from build123d import *

# Parameters (mm, degrees)
F1_DEPTH = 5.1
F2_W     = 3.2
F2_H     = 3.2
F4_DEPTH = 11
F3_W     = 3.2
F3_H     = 3.2
F5_DEPTH = 11
F6_DEPTH = 1


# Not quite as in the source:
# - a feature names something its author has since deleted; it is built from what else it names


with BuildPart() as f1:
    # F0 (on Top) → F1 (new body)
    with BuildSketch(Plane.XY):
        Polygon((-17.8524617243, -0.2032842353), (-25.3224617243, -0.2032842353), (-25.3224617243, -13.2032842353), (-5.3224617243, -13.2032842353), (-5.3224617243, -0.2032842353), (-12.7924617243, -0.2032842353), (-12.7924617243, -8.0232842353), (-11.6424617243, -8.0232842353), (-11.6424617243, -10.1232842353), (-19.0024617243, -10.1232842353), (-19.0024617243, -8.0232842353), (-17.8524617243, -8.0232842353), align=None)
    extrude(amount=F1_DEPTH)

    # F2 (on face) → F4 (cut)
    with BuildSketch(Plane(origin=(0, -0.2032842353, 0), x_dir=(-1, 0, 0), z_dir=(0, 1, 0))):
        with Locations((9.6924617243, 2.55)):
            Rectangle(F2_W, F2_H)
    extrude(amount=-F4_DEPTH, mode=Mode.SUBTRACT)

    # F3 (on face) → F5 (cut)
    with BuildSketch(Plane(origin=(0, -0.2032842353, 0), x_dir=(-1, 0, 0), z_dir=(0, 1, 0))):
        with Locations((20.9524617243, 2.55)):
            Rectangle(F3_W, F3_H)
    extrude(amount=-F5_DEPTH, mode=Mode.SUBTRACT)

    # F6 (cut): a face of the model
    f6_faces = [f1.faces().sort_by_distance(p)[0] for p in [
        (-19.2409989331, -9.0732842353, 5.1),
    ]]
    extrude(f6_faces, amount=-F6_DEPTH, mode=Mode.SUBTRACT)


solid = f1.part
Geometry check sheet. Reference: the model listing, model coordinates, mm. A direction names the side the tool comes from. Coordinates: 2 decimals unless noted, no trailing zeros. Order: outer loops, then holes, each group sorted by start corner. A loop starts at its lowest first (then second) coordinate and runs counter-clockwise, first axis right, second up. Notation, with made-up numbers: M 64.25,27.25 L 77.25,27.25 A26 cw 77.25,65.25 Z; hole C -22.5,-16.75 d11. An arc over 180 degrees is marked long. Use CSV: the item, a comma, the result in double quotes.
Item 1: Thickness scan on line 1 along X through (y, z) = (-4, 1.8); line 2 along X through (y, z) = (-10, 2.1); line 3 along X through (y, z) = (-4.75, 0.4). Record the ranges inside material, lowest first.
Returned:
line 1,"x = -25.32 to -22.55, -19.35 to -17.85, -12.79 to -11.29, -8.09 to -5.32"
line 2,"x = -25.32 to -22.55, -19.35 to -19, -11.64 to -11.29, -8.09 to -5.32"
line 3,"x = -25.32 to -17.85, -12.79 to -5.32"
Item 2: Tool access check on faces 5 (the flat face through (-5.322, -7, 2)), 6 (the flat face through (-12, -8.023, 2)), 7 (the flat face through (-22.552, -6, 3)), 8 (the flat face through (-12.792, -4, 2)). Record the directions out of +Z, -Z, +X, -X, +Y, -Y that give a thin tool (end or side, any length) a straight path to the whole face; none if there is none.
Returned:
face 5,"+Z, -Z, +X, +Y, -Y"
face 6,"+Z, -Z"
face 7,"+Z, +Y"
face 8,"+Z, -Z, +Y"
Item 3: Mould release check, pull along X, two halves, no side actions. Record for faces 1 (the flat face through (-10, -6, 0.95)), 2 (the flat face through (-11.292, -6, 3)), 3 (the flat face through (-25.322, -7, 2)), 4 (the flat face through (-18.3, -7.2, 4.1)): pulls with the +X half, pulls with the -X half, needs draft (parallel to the pull), parting line crosses it, or undercut.
Returned:
face 1,"undercut"
face 2,"undercut"
face 3,"pulls with the -X half"
face 4,"needs draft"
Item 4: Cross-section at C-C on z = 3.75. Record the cut outline in (x, y), then the cut area to 3 significant figures.
Returned:
outline,"M -25.32,-13.2 L -5.32,-13.2 L -5.32,-0.2 L -8.09,-0.2 L -8.09,-11.2 L -11.29,-11.2 L -11.29,-0.2 L -12.79,-0.2 L -12.79,-8.02 L -11.64,-8.02 L -11.64,-10.12 L -19,-10.12 L -19,-8.02 L -17.85,-8.02 L -17.85,-0.2 L -19.35,-0.2 L -19.35,-11.2 L -22.55,-11.2 L -22.55,-0.2 L -25.32,-0.2 Z"
area,"135 mm2"
Item 5: Cross-section at D-D on y = -9.5. Record the cut outline in (x, z), then the cut area to 3 significant figures.
Returned:
outline,"M -25.32,0 L -19,0 L -19,4.1 L -19.35,4.1 L -19.35,0.95 L -22.55,0.95 L -22.55,4.1 L -25.32,4.1 Z; M -11.64,0 L -5.32,0 L -5.32,4.1 L -8.09,4.1 L -8.09,0.95 L -11.29,0.95 L -11.29,4.1 L -11.64,4.1 Z"
area,"31.7 mm2"
Item 6: Cross-section at A-A on x = -18.75. Record the cut outline in (y, z), then the cut area to 3 significant figures.
Returned:
outline,"M -13.2,0 L -10.12,0 L -10.12,4.1 L -13.2,4.1 Z; M -8.02,0 L -0.2,0 L -0.2,4.1 L -8.02,4.1 Z"
area,"44.7 mm2"
Item 7: Cross-section at B-B on y = -4.25. Record the cut outline in (x, z), then the cut area to 3 significant figures.
Returned:
outline,"M -25.32,0 L -17.85,0 L -17.85,4.1 L -19.35,4.1 L -19.35,0.95 L -22.55,0.95 L -22.55,4.1 L -25.32,4.1 Z; M -12.79,0 L -5.32,0 L -5.32,4.1 L -8.09,4.1 L -8.09,0.95 L -11.29,0.95 L -11.29,4.1 L -12.79,4.1 Z"
area,"41.1 mm2"
Item 8: Gauge pin test, flat ends, axial feed: pin 1 Ø1.6 at (x, y) = (-21.5, -4) entering from +Z; pin 2 Ø1.2 at (x, z) = (-15.5, 1) entering from +Y; pin 3 Ø0.9 at (x, z) = (-9, 2) entering from +Y. Record the tip position at first contact, or that the pin passes through.
Returned:
pin 1,"stops at z = 0.95"
pin 2,"stops at y = -10.12"
pin 3,"stops at y = -11.2"
